from build123d import *

# Parameters (mm, degrees)
F0_W     = 63.5
F0_H     = 25.4
F1_DEPTH = 19.05
F2_R     = 6.35
F3_DEPTH = 25.4
F4_R     = 12.69999
F5_SIZE  = 1.5875


# Not quite as in the source:
# - a fillet or chamfer is up to 0.001 mm smaller than in the source, because OpenCascade refuses the exact size


with BuildPart() as f1:
    # F0 (on Right) → F1 (new body)
    with BuildSketch(Plane.YZ):
        Rectangle(F0_W, F0_H)
    extrude(amount=F1_DEPTH)

    # F2 (on face) → F3 (cut)
    with BuildSketch(Plane.YZ.offset(19.05)):
        with Locations((19.05, 0)):
            Circle(F2_R)
    extrude(amount=-F3_DEPTH, mode=Mode.SUBTRACT)

    # F4 (radius 12.7 in the source; OpenCascade refuses exactly that, so slightly less here)
    f4_edges = [f1.edges().sort_by_distance(p)[0] for p in [
        (9.525, 31.75, 12.7),
        (9.525, 31.75, -12.7),
    ]]
    fillet(f4_edges, radius=F4_R)

    # F5
    f5_edges = [f1.edges().sort_by_distance(p)[0] for p in [
        (9.525, -31.75, 12.7),
        (9.525, -31.75, -12.7),
    ]]
    chamfer(f5_edges, length=F5_SIZE)


solid = f1.part
Geometry check sheet. Reference: the model listing, model coordinates, mm. Round coordinates to 2 decimals unless told otherwise and drop trailing zeros. Write each loop counter-clockwise with the first axis right and the second up, starting at its lowest first coordinate (ties: lowest second). Pieces come first, ordered by that corner, then holes.
Item 1: Section check A-A (z = -2.5). Record the boundary of the cut face in (x, y).
Determined:
outline: (0, -31.75) - (19.05, -31.75) - (19.05, 13.21) - (0, 13.21) - close; (0, 24.89) - (19.05, 24.89) - (19.05, 31.5) - (0, 31.5) - close
Item 2: Mould release check, pull along Z, two halves, no side actions. Record for faces 1 (the face through (9.392, -30.967, -11.895)), 2 (the face through (9.392, -30.945, 11.917)), 3 (the face through (19.05, 0, 0)), 4 (the face through (9.658, 24.916, -2.432)): +Z half, -Z half, draft (parallel to the pull), parting line (faces both ways), or undercut.
Determined:
face 1: -Z half
face 2: +Z half
face 3: draft
face 4: undercut
Item 3: Material ranges on line 1 along Z through (x, y) = (14.75, 19.05); line 2 along Y through (x, z) = (2.25, 5.25); line 3 along Y through (x, z) = (10.5, -4.5), recorded low to high.
Determined:
line 1: z = -12.7 to -6.35, 6.35 to 12.7
line 2: y = -31.75 to 15.48, 22.62 to 30.61
line 3: y = -31.75 to 14.57, 23.53 to 30.93
Item 4: Section check D-D (z = -7). Record the boundary of the cut face in (x, y), plus the area to 3 significant figures.
Determined:
outline: (0, -31.75) - (19.05, -31.75) - (19.05, 29.65) - (0, 29.65) - close
area: 1,170 mm2
Item 5: Section check C-C (y = 14.5). Record the boundary of the cut face in (x, z), plus the area to 3 significant figures.
Determined:
outline: (0, -12.7) - (19.05, -12.7) - (19.05, -4.43) - (0, -4.43) - close; (0, 4.43) - (19.05, 4.43) - (19.05, 12.7) - (0, 12.7) - close
area: 315 mm2
Item 6: Go/stop test with flat-tipped pins: pin 1 Ø11.5 at (y, z) = (19.05, 0) entering from +X; pin 2 Ø1.5 at (x, z) = (16, 4.5) entering from +Y; pin 3 Ø1 at (x, z) = (4.5, 3) entering from +Y. Record where each tip stops, or that it passes through.
Determined:
pin 1: passes through
pin 2: stops at y = 31.18
pin 3: stops at y = 31.5
